Work out the finished part from the listing and answer in its coordinate system (mm). A direction names the side the tool comes from. Coordinates: 2 decimals unless noted, no trailing zeros. Order: outer loops, then holes, each group sorted by start corner. A loop starts at its lowest first (then second) coordinate and runs counter-clockwise, first axis right, second up. Notation, with made-up numbers: (19.25, -10) - (31.25, -10) arc R19 cw to (31.25, 24) - close; hole circle Ø3 at (-23, 5). An arc over 180 degrees is marked (long way). Answer as a JSON object with one key per item and string values. Group by question number.
1) A tool of negligible diameter and unlimited length cuts with its end or side. For faces 1 (the face through (0, -5.5, -1)), 2 (the face through (0, 7, 5)), 3 (the face through (0, 5, 3)), 4 (the face through (-5, 7, 3)), 5 (the face through (-6, -7, -1)), from which of +Z, -Z, +X, -X, +Y, -Y can it reach the whole face along a straight path? Write none if from no direction.
2) Section B-B (z = 8) is taken. Give the vertices of the cut face in (x, y), plus the area to 3 significant figures.
3) Each of these flat-tipped pins is pushed along its axis until it touches: P1, Ø2, axis at y = -8.5, z = -1.5, coming from the -X side; P2, Ø5, axis at y = -1.5, z = 11, coming from the -X side; P3, Ø1, axis at x = -0.5, z = -1, coming from the +Y side. Where does it stop, or does it pass through?
4) Section A-A (y = 0) is taken. Give the vertices of the cut face in (x, z), plus the area to 3 significant figures.
5) Find the intervals of material crossed by line 1 along Z through (x, y) = (-15, -6); line 2 along Z through (x, y) = (1, -6); line 3 along X through (y, z) = (-1.5, 5.5), in increasing order.
6) Section C-C (x = 1) is taken. Give the vertices of the cut face in (y, z).
7) The mould has two halves that part along X. Classify faces 6 (the face through (22.5, 0, 1)), 7 (the face through (0, 0, 1.6)), 8 (the face through (-21.5, 0, -1)): released by +X, released by -X, zero draft, split by the parting line, or undercut.
8) Section D-D (x = -13) is taken. Give the vertices of the cut face in (y, z), plus the area to 3 significant figures.
from build123d import *

# Parameters (mm, degrees)
SKETCH_1_W          = 45
SKETCH_1_H          = 20
EXTRUDE_1_DEPTH     = 1.6
SKETCH_2_R          = 8
EXTRUDE_2_DEPTH     = 11.7
FILLET_1_R          = 0.5
SKETCH_3_R          = 6
CUT_EXTRUDE_1_DEPTH = 0.5
EXTRUDE_3_DEPTH     = 3.4
SKETCH_5_W          = 10
SKETCH_5_H          = 2.5
EXTRUDE_4_DEPTH     = 2
EXTRUDE_5_DEPTH     = 1.6


with BuildPart() as part:
    # Эскиз1 → Бобышка-Вытянуть1 (new body)
    with BuildSketch(Plane.XY):
        Rectangle(SKETCH_1_W, SKETCH_1_H)
    extrude(amount=EXTRUDE_1_DEPTH)

    # Эскиз2 → Бобышка-Вытянуть2 (add)
    with BuildSketch(Plane.XY.offset(1.6)):
        with Locations(Location((-13, 0, 0), (0, 0, 180))):
            Circle(SKETCH_2_R)
        with Locations(Location((13, 0, 0), (0, 0, 180))):
            Circle(SKETCH_2_R)
    extrude(amount=EXTRUDE_2_DEPTH)

    # Скругление1
    fillet_1_edges = [part.edges().sort_by_distance(p)[0] for p in [
        (-5, 0, 13.3),
        (21, 0, 13.3),
    ]]
    fillet(fillet_1_edges, radius=FILLET_1_R)

    # Эскиз3 → Вырез-Вытянуть1 (cut)
    with BuildSketch(Plane.XY.offset(13.3)):
        with Locations((-13, 0)):
            Circle(SKETCH_3_R)
        with Locations((13, 0)):
            Circle(SKETCH_3_R)
    extrude(amount=-CUT_EXTRUDE_1_DEPTH, mode=Mode.SUBTRACT)

    # Эскиз4 → Бобышка-Вытянуть3 (add)
    with BuildSketch(Plane.XY.offset(1.6)):
        with BuildLine():
            Line((-3, 9), (3, 9))
            ThreePointArc((3, 9), (5, 7), (3, 5))
            Line((3, 5), (-3, 5))
            ThreePointArc((-3, 5), (-5, 7), (-3, 9))
        make_face()
    extrude(amount=EXTRUDE_3_DEPTH)

    # Эскиз5 → Бобышка-Вытянуть4 (add)
    with BuildSketch(Plane(origin=(0, 0, 0), x_dir=(-1, 0, 0), z_dir=(0, 0, -1))):
        with Locations((0, -7.75)):
            Rectangle(SKETCH_5_W, SKETCH_5_H)
    extrude(amount=EXTRUDE_4_DEPTH)

    # Эскиз8 → Бобышка-Вытянуть5 (add)
    with BuildSketch(Plane(origin=(0, 0, 0), x_dir=(-1, 0, 0), z_dir=(0, 0, -1))):
        Polygon((-6, -9), (-6, -5.5), (6, -5.5), (6, -9), (21.5, -9), (21.5, 9), (-21.5, 9), (-21.5, -9), align=None)
    extrude(amount=EXTRUDE_5_DEPTH)


solid = part.part
Report:
{
 "1": {"face 1": "-Z", "face 2": "+Z, +Y, -Y", "face 3": "+Z, -Y", "face 4": "+Z", "face 5": "-Z, -Y"},
 "2": {"outline": "circle Ø16 at (-13, 0); circle Ø16 at (13, 0)", "area": "402 mm²"},
 "3": {"P1": "stops at x = -21.5", "P2": "stops at x = -21", "P3": "stops at y = 9"},
 "4": {"outline": "(-22.5, 0) - (-21.5, 0) - (-21.5, -1.6) - (21.5, -1.6) - (21.5, 0) - (22.5, 0) - (22.5, 1.6) - (21, 1.6) - (21, 12.8) arc R0.5 ccw to (20.5, 13.3) - (19, 13.3) - (19, 12.8) - (7, 12.8) - (7, 13.3) - (5.5, 13.3) arc R0.5 ccw to (5, 12.8) - (5, 1.6) - (-5, 1.6) - (-5, 12.8) arc R0.5 ccw to (-5.5, 13.3) - (-7, 13.3) - (-7, 12.8) - (-19, 12.8) - (-19, 13.3) - (-20.5, 13.3) arc R0.5 ccw to (-21, 12.8) - (-21, 1.6) - (-22.5, 1.6) - close", "area": "503 mm²"},
 "5": {"line 1": "z = -1.6 to 13.3", "line 2": "z = 0 to 1.6", "line 3": "x = -20.86 to -5.14, 5.14 to 20.86"},
 "6": {"outline": "(-10, 0) - (-9, 0) - (-9, -2) - (-6.5, -2) - (-6.5, 0) - (-5.5, 0) - (-5.5, -1.6) - (9, -1.6) - (9, 0) - (10, 0) - (10, 1.6) - (9, 1.6) - (9, 5) - (5, 5) - (5, 1.6) - (-10, 1.6) - close"},
 "7": {"face 6": "released by +X", "face 7": "undercut", "face 8": "released by -X"},
 "8": {"outline": "(-10, 0) - (-9, 0) - (-9, -1.6) - (9, -1.6) - (9, 0) - (10, 0) - (10, 1.6) - (8, 1.6) - (8, 12.8) arc R0.5 ccw to (7.5, 13.3) - (6, 13.3) - (6, 12.8) - (-6, 12.8) - (-6, 13.3) - (-7.5, 13.3) arc R0.5 ccw to (-8, 12.8) - (-8, 1.6) - (-10, 1.6) - close", "area": "242 mm²"}
}
